```python
from build123d import *

# Parameters (mm, degrees)
SKETCH1_R           = 14.7701
SKETCH1_R_2         = 13.3223
BOSS_EXTRUDE1_DEPTH = 2032
SKETCH2_R           = 3.175
CUT_EXTRUDE1_DEPTH  = 2033.107357328


with BuildPart() as part:
    # Sketch1 → Boss-Extrude1 (new body)
    with BuildSketch(Plane(origin=(0, 0, 0), x_dir=(0, 0, -1), z_dir=(1, 0, 0))):
        Circle(SKETCH1_R)
        Circle(SKETCH1_R_2, mode=Mode.SUBTRACT)
    extrude(amount=BOSS_EXTRUDE1_DEPTH)

    # Sketch2 → Cut-Extrude1 (cut, symmetric)
    with BuildSketch(Plane.XY):
        with Locations((19.05, 0)):
            Circle(SKETCH2_R)
        with Locations((44.45, 0)):
            Circle(SKETCH2_R)
    cut_extrude1 = extrude(amount=CUT_EXTRUDE1_DEPTH, both=True, mode=Mode.SUBTRACT)

    # Mirror1: Cut-Extrude1 across plane
    add(cut_extrude1.mirror(Plane(origin=(1016, 0, 0), x_dir=(0, 0, 1), z_dir=(1, 0, 0))), mode=Mode.SUBTRACT)


solid = part.part
```
Source: CAD feature listing. Evaluate the final solid. Frame: model axes, mm. Round coordinates to 2 decimals unless told otherwise and drop trailing zeros. Write each loop counter-clockwise with the first axis right and the second up, starting at its lowest first coordinate (ties: lowest second). Pieces come first, ordered by that corner, then holes. Notation, with made-up numbers: M 20,-22.75 L 40,-22.75 A19 ccw 40,-17.75 Z; hole C -2.5,74 d7. An arc over 180 degrees is marked long. Answer as a JSON object with one key per item and string values. Group by question number.
(1) First-contact query: pin 1 (12 mm diameter, centred on x = 1508.5, y = -7, fed in from -Z); pin 2 (16 mm diameter, centred on y = 0, z = 0, fed in from +X); pin 3 (3 mm diameter, centred on x = 633, y = -7.5, fed in from -Z); pin 4 (1 mm diameter, centred on x = 695, y = 4.5, fed in from -Z). Flat tips, straight axial feed; report the tip coordinate or a pass-through.
(2) Section query B-B on x = 147.5. Output: boundary loops of the cut face in (y, z), then the cut area to 3 significant figures.
(3) Section query A-A on z = 0. Output: boundary loops of the cut face in (x, y), then the cut area to 3 significant figures.
(4) Ray query, line 1 (X direction, y = 0, z = -13.5) (3 decimals); line 2 (Y direction, x = 773.5, z = 3); line 3 (Z direction, x = 1046, y = -2.75). Return the intervals inside material, ascending. Write a range as [from, to].
Computed values:
{
 "1": {"pin 1": "z = -14.74", "pin 2": "through", "pin 3": "z = -13.5", "pin 4": "z = -14.22"},
 "2": {"outline": "C 0,0 d29.54; hole C 0,0 d26.64", "area": "128 mm^2"},
 "3": {"outline": "M 0,-14.77 L 2032,-14.77 L 2032,-13.32 L 0,-13.32 Z; M 0,13.32 L 2032,13.32 L 2032,14.77 L 0,14.77 Z", "area": "5,880 mm^2"},
 "4": {"line 1": "[0, 15.875], [22.225, 41.275], [47.625, 1984.375], [1990.725, 2009.775], [2016.125, 2032]", "line 2": "[-14.46, -12.98], [12.98, 14.46]", "line 3": "[-14.51, -13.04], [13.04, 14.51]"}
}
